Autodesk Inventor part; units mm, degrees
ref_plane "YZ Plane" through (0, 0, 0) normal (1, 0, 0) x (0, 1, 0)
ref_plane "XZ Plane" through (0, 0, 0) normal (0, 1, 0) x (-1, 0, 0)
ref_plane "XY Plane" through (0, 0, 0) normal (0, 0, 1) x (1, 0, 0)
sketch "Sketch1" plane through (0, 0, 0) normal (0, 0, 1) x (1, 0, 0)
  line L0 (0, 0) -> (190.5, 0) construction
  line L1 (0, -19.05) -> (190.5, -19.05)
  line L2 (190.5, 19.05) -> (0, 19.05)
  arc A0 (0, 19.05) -> (0, -19.05) centre (0, 0) ccw
  arc A1 (190.5, -19.05) -> (190.5, 19.05) centre (190.5, 0) ccw
  circle A2 centre (0, 0) radius 3.175
  circle A3 centre (190.5, 0) radius 3.175
  point P0 (95.25, 0)
  dimension "d0" = 190.5
  dimension "d1" = 38.1
  dimension "d2" = 6.35
extrude "Extrusion1" add sketch "Sketch1" along normal blind 2.54
properties part number "link"
Build history of the part. All positions in model axes, mm. Give positions to 0.01 mm unless a question says otherwise; leave off trailing zeros. Loops run counter-clockwise (first coordinate to the right, second up) from the corner with the lowest first, then second, coordinate; pieces in that order, holes last. Notation, with made-up numbers: (2, 14.5) - (15, 14.5) arc R26 cw to (15, 44.5) - close; hole circle Ø6 at (39.5, 25.5). An arc over 180 degrees is marked (long way). Use a Markdown table: item, result.
(1) Band-saw the part on A-A (z = 2). Give the cut face in (x, y) (3 decimals).
Taken from the geometry:
| item | result |
|---|---|
| outline | (0, -19.05) - (190.5, -19.05) arc R19.05 ccw to (190.5, 19.05) - (0, 19.05) arc R19.05 ccw to start; hole circle Ø6.35 at (0, 0); hole circle Ø6.35 at (190.5, 0) |
(2) Wall check: line 1 along Y through (x, z) = (190.5, 0.65) (3 decimals); line 2 along Y through (x, z) = (190, 1); line 3 along X through (y, z) = (-2, 1.9). Give the ranges that are in metal, low to high.
Taken from the geometry:
| item | result |
|---|---|
| line 1 | -19.05 to -3.175, 3.175 to 19.05 |
| line 2 | -19.05 to -3.14, 3.14 to 19.05 |
| line 3 | -18.94 to -2.47, 2.47 to 188.03, 192.97 to 209.44 |
(3) Band-saw the part on B-B (y = 0). Give the cut face in (x, z) (3 decimals), and give its area (3 significant figures).
Taken from the geometry:
| item | result |
|---|---|
| outline | (-19.05, 0) - (-3.175, 0) - (-3.175, 2.54) - (-19.05, 2.54) - close; (3.175, 0) - (187.325, 0) - (187.325, 2.54) - (3.175, 2.54) - close; (193.675, 0) - (209.55, 0) - (209.55, 2.54) - (193.675, 2.54) - close |
| area | 548 mm2 |
(4) Drop flat-ended pins along their axis: pin 1 Ø2 at (x, y) = (22, -3) entering from -Z; pin 2 Ø4 at (x, y) = (0, 0) entering from +Z; pin 3 Ø1.5 at (y, z) = (-2, 2) entering from -X. Give the stop position or say it passes through.
Taken from the geometry:
| item | result |
|---|---|
| pin 1 | z = 0 |
| pin 2 | through |
| pin 3 | x = -19.01 |
